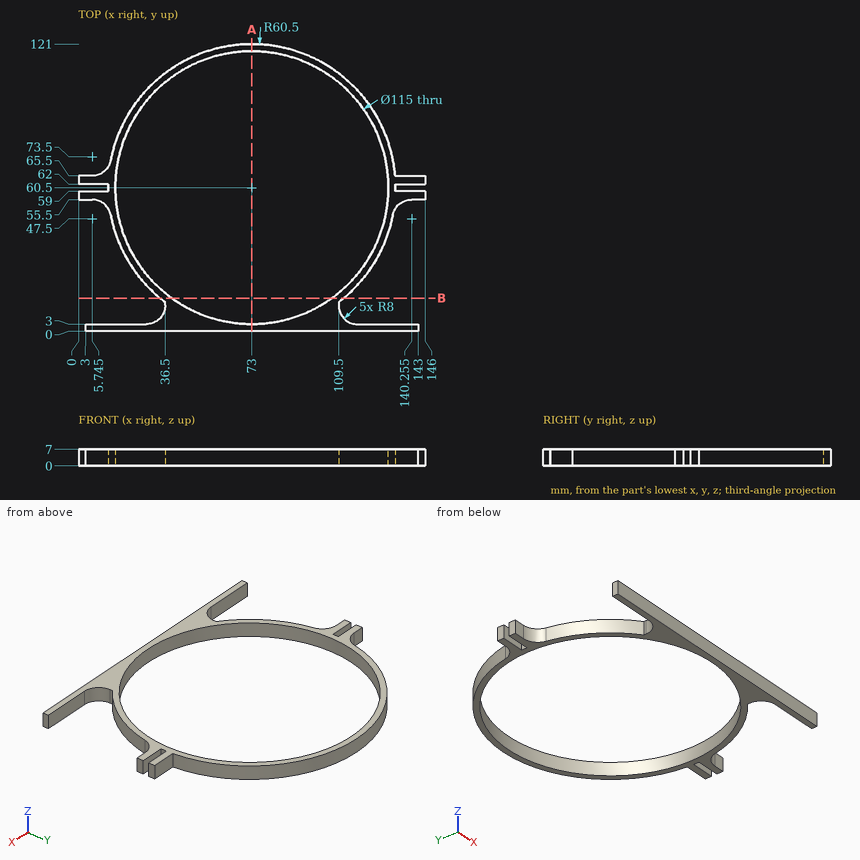
Check sheet for the drawn part. Datum: minimum x, y, z corner. Units: mm. Give positions to 0.01 mm unless a question says otherwise; leave off trailing zeros. Order: outer loops, then holes, each group sorted by start corner. A loop starts at its lowest first (then second) coordinate and runs counter-clockwise, first axis right, second up. Notation, with made-up numbers: (70, 63) - (126, 63) arc R15 cw to (126, 90) - close; hole circle Ø9 at (87, 9). An arc over 180 degrees is marked (long way). Answer in a Markdown table with one row per item. Add a question column.
Q1. Cross-section at A-A, the plane x = 73. Enter the section's corners in (y, z).
Q2. Material ranges on probe 1 along Y at (x, z) = (140.5, 6.5); probe 2 along Y at (x, z) = (72, 5.25); probe 3 along X at (y, z) = (60.5, 4.5), recorded low to high. Write a range as from..to.
Q3. Cross-section at B-B, the plane y = 14. Enter the section's corners in (x, z).
Q4. Gauge pin test, flat ends, axial feed: pin 1 (4 mm diameter, centred on x = 129, z = 2.5, fed in from +Y); pin 2 (0.9 mm diameter, centred on y = 1, z = 4, fed in from +X); pin 3 (1.4 mm diameter, centred on y = 12, z = 3, fed in from -X). Record the tip position at first contact, or that the pin passes through.
Check values:
| question | item | result |
|---|---|---|
| 1 | outline | (0, 0) - (3, 0) - (3, 7) - (0, 7) - close; (118, 0) - (121, 0) - (121, 7) - (118, 7) - close |
| 2 | probe 1 | y = 0..3, 55.5..59, 62..65.5 |
| 2 | probe 2 | y = 0..3.01, 117.99..120.99 |
| 2 | probe 3 | x = 12.5..15.5, 130.5..133.5 |
| 3 | outline | (34.3, 0) - (39.18, 0) - (39.18, 7) - (34.3, 7) - close; (106.82, 0) - (111.7, 0) - (111.7, 7) - (106.82, 7) - close |
| 4 | pin 1 | stops at y = 87.78 |
| 4 | pin 2 | stops at x = 143 |
| 4 | pin 3 | stops at x = 35.91 |
